Input: dimensioned drawing with shaded views. Units: mm. Origin: part minimum x, y, z. Round coordinates to 2 decimals unless told otherwise and drop trailing zeros. Loops run counter-clockwise (first coordinate to the right, second up) from the corner with the lowest first, then second, coordinate; pieces in that order, holes last. Notation, with made-up numbers: M 62,59 L 119,59 A18 ccw 119,66 Z; hole C -12.75,-37 d7. An arc over 180 degrees is marked long. Return JSON: item names as keys, results as strings.
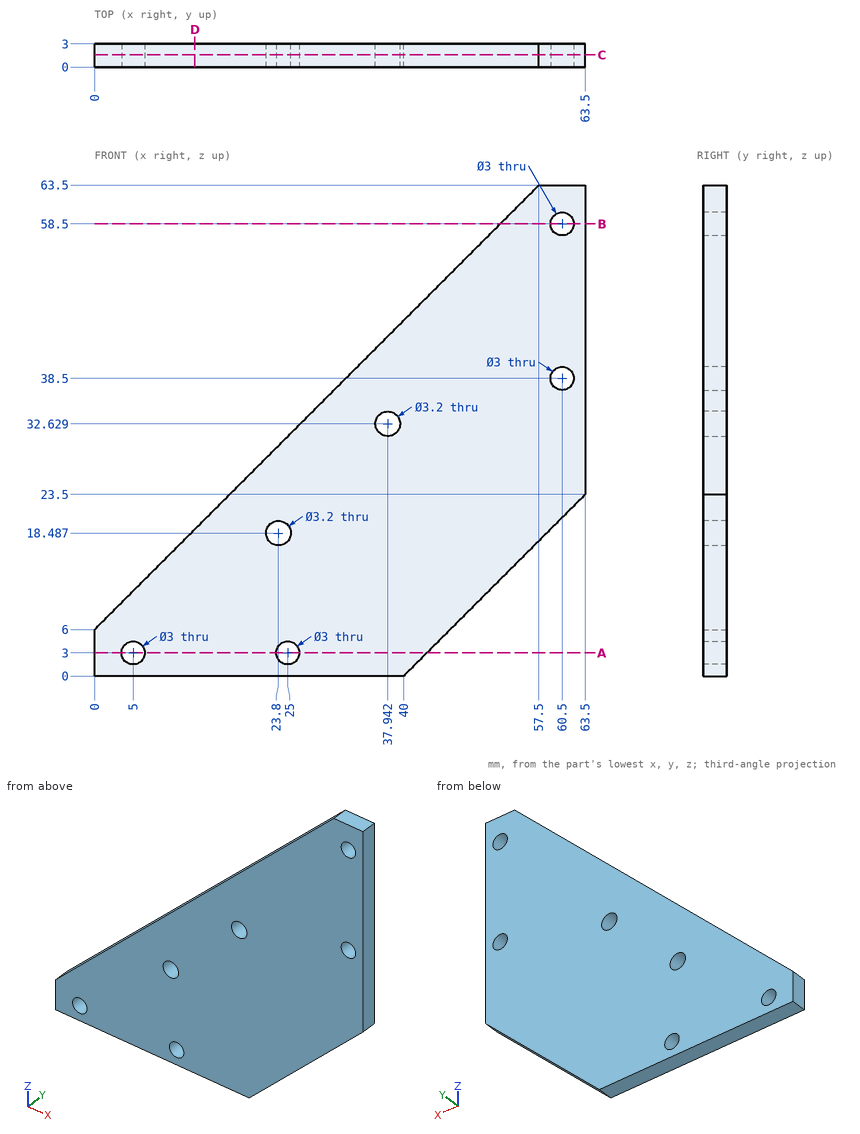
Q1. Section query B-B (z = 58.5). Output: boundary loops of the cut face in (x, y), plus the area to 3 significant figures.
Determined:
{"outline": "M 52.5,0 L 59,0 L 59,3 L 52.5,3 Z; M 62,0 L 63.5,0 L 63.5,3 L 62,3 Z", "area": "24.0 mm^2"}
Q2. Section query D-D (x = 13). Output: boundary loops of the cut face in (y, z).
Determined:
{"outline": "M 0,0 L 3,0 L 3,19 L 0,19 Z"}
Q3. Section query C-C (y = 1.6). Output: boundary loops of the cut face in (x, z), plus the area to 3 significant figures.
Determined:
{"outline": "M 0,0 L 40,0 L 63.5,23.5 L 63.5,63.5 L 57.5,63.5 L 0,6 Z; hole C 5,3 d3; hole C 23.8,18.49 d3.2; hole C 25,3 d3; hole C 37.94,32.63 d3.2; hole C 60.5,38.5 d3; hole C 60.5,58.5 d3", "area": "2,060 mm^2"}
Q4. Material intervals for L1, parallel to Z at x = 60.5, y = 1.3; L2, parallel to X at y = 1.35, z = 3; L3, parallel to X at y = 0.9, z = 32 (1 decimal), sorted ascending.
Determined:
{"L1": "z = 20.5 to 37, 40 to 57, 60 to 63.5", "L2": "x = 0 to 3.5, 6.5 to 23.5, 26.5 to 43", "L3": "x = 26 to 36.5, 39.4 to 63.5"}
Q5. Pin query (flat end, axial travel): pin 1 (1.9 mm diameter, centred on x = 37.94, z = 32.63, fed in from -Y); pin 2 (1 mm diameter, centred on x = 28, y = 2, fed in from +Z); pin 3 (1.5 mm diameter, centred on y = 1.5, z = 9, fed in from -X). Return the tip coordinate at first contact, or that it passes through.
Determined:
{"pin 1": "passes through", "pin 2": "stops at z = 34.5", "pin 3": "stops at x = 2.25"}
Q6. Section query A-A (z = 3). Output: boundary loops of the cut face in (x, y).
Determined:
{"outline": "M 0,0 L 3.5,0 L 3.5,3 L 0,3 Z; M 6.5,0 L 23.5,0 L 23.5,3 L 6.5,3 Z; M 26.5,0 L 43,0 L 43,3 L 26.5,3 Z"}
